from build123d import *

# Parameters (mm, degrees)
F0_W     = 28.35
F0_H     = 108.95
F0_W_2   = 6
F0_H_2   = 28
F0_W_3   = 4
F0_H_3   = 32.75
F0_H_4   = 9.8
F0_H_5   = 24
F0_W_4   = 9.65
F0_H_6   = 76.2
F0_H_7   = 11.1
F0_R     = 3
F1_DEPTH = 1


# Not quite as in the source:
# - a feature names something its author has since deleted; it is built from what else it names


with BuildPart() as f1:
    # F0 (on Right) → F1 (new body)
    with BuildSketch(Plane.YZ):
        Polygon((178.337747033, -16.9212994559), (149.987747033, -16.9212994559), (130.337747033, -16.9212994559), (130.337747033, -39.6712994559), (251.987747033, -39.6712994559), (251.987747033, -16.9212994559), (182.337747033, -16.9212994559), align=None)
        with Locations((164.162747033, 37.5537005441)):
            Rectangle(F0_W, F0_H)
        Polygon((130.337747033, -16.9212994559), (149.987747033, -16.9212994559), (149.987747033, 92.0287005441), (148.337747033, 92.0287005441), (136.337747033, 92.0287005441), (136.337747033, 68.0287005441), (136.337747033, 56.9287005441), (136.337747033, 28.9287005441), (136.337747033, 19.1287005441), (136.337747033, -8.8712994559), (130.337747033, -8.8712994559), align=None)
        Polygon((130.337747033, -39.6712994559), (130.337747033, -16.9212994559), (110.687747033, -16.9212994559), (82.337747033, -16.9212994559), (82.337747033, -28.2962994559), (82.337747033, -39.6712994559), align=None)
        Polygon((110.687747033, -16.9212994559), (130.337747033, -16.9212994559), (130.337747033, -8.8712994559), (124.337747033, -8.8712994559), (124.337747033, 19.1287005441), (124.337747033, 21.9287005441), (124.337747033, 24.7287005441), (124.337747033, 27.5287005441), (124.337747033, 28.9287005441), (124.337747033, 56.9287005441), (130.337747033, 56.9287005441), (130.337747033, 68.0287005441), (124.337747033, 68.0287005441), (124.337747033, 92.0287005441), (130.337747033, 92.0287005441), (136.337747033, 92.0287005441), (148.337747033, 92.0287005441), (148.337747033, 102.1287005441), (148.337747033, 105.1287005441), (143.337747033, 105.1287005441), (130.337747033, 105.1287005441), (112.337747033, 105.1287005441), (112.337747033, 102.1287005441), (112.337747033, 92.0287005441), (110.687747033, 92.0287005441), align=None)
        Polygon((178.337747033, 92.0287005441), (178.337747033, -16.9212994559), (182.337747033, -16.9212994559), (182.337747033, 92.0287005441), (179.8798441887, 92.0287005441), align=None)
        Polygon((82.337747033, -16.9212994559), (110.687747033, -16.9212994559), (110.687747033, 92.0287005441), (82.337747033, 92.0287005441), (82.337747033, 15.8287005441), align=None)
        with Locations((133.337747033, 5.1287005441)):
            Rectangle(F0_W_2, F0_H_2)
        with Locations((127.337747033, 5.1287005441)):
            Rectangle(F0_W_2, F0_H_2)
        Polygon((182.337747033, 92.0287005441), (182.337747033, -16.9212994559), (251.987747033, -16.9212994559), (251.987747033, 92.0287005441), (226.687747033, 92.0287005441), (216.162747033, 92.0287005441), (214.687747033, 92.0287005441), align=None)
        Polygon((82.337747033, -28.2962994559), (82.337747033, -16.9212994559), (78.337747033, -16.9212994559), (68.687747033, -16.9212994559), (68.687747033, -28.2962994559), align=None)
        with Locations((80.337747033, -0.5462994559)):
            Rectangle(F0_W_3, F0_H_3)
        with Locations((133.337747033, 24.0287005441)):
            Rectangle(F0_W_2, F0_H_4)
        Polygon((124.337747033, 19.1287005441), (130.337747033, 19.1287005441), (130.337747033, 28.9287005441), (124.337747033, 28.9287005441), (124.337747033, 27.5287005441), (124.337747033, 24.7287005441), (124.337747033, 21.9287005441), align=None)
        Polygon((60.012747033, -39.6712994559), (82.337747033, -39.6712994559), (82.337747033, -28.2962994559), (68.687747033, -28.2962994559), (63.512747033, -28.2962994559), (60.012747033, -28.2962994559), align=None)
        with Locations((133.337747033, 80.0287005441)):
            Rectangle(F0_W_2, F0_H_5)
        with Locations((73.512747033, -0.5462994559)):
            Rectangle(F0_W_4, F0_H_3)
        with Locations((80.337747033, 53.9287005441)):
            Rectangle(F0_W_3, F0_H_6)
        with Locations((133.337747033, 42.9287005441)):
            Rectangle(F0_W_2, F0_H_2)
        with Locations((127.337747033, 42.9287005441)):
            Rectangle(F0_W_2, F0_H_2)
        with Locations((127.337747033, 80.0287005441)):
            Rectangle(F0_W_2, F0_H_5)
        with Locations((133.337747033, 62.4787005441)):
            Rectangle(F0_W_2, F0_H_7)
        with BuildLine():
            Line((68.687747033, -28.2962994559), (68.687747033, -16.9212994559))
            Line((68.687747033, -16.9212994559), (68.687747033, 15.8287005441))
            Line((68.687747033, 15.8287005441), (54.687747033, 15.8287005441))
            Line((54.687747033, 15.8287005441), (44.512747033, 15.8287005441))
            Line((44.512747033, 15.8287005441), (37.687747033, 15.8287005441))
            Line((37.687747033, 15.8287005441), (8.687747033, 15.8287005441))
            Line((8.687747033, 15.8287005441), (8.687747033, -28.2962994559))
            Line((8.687747033, -28.2962994559), (25.512747033, -28.2962994559))
            ThreePointArc((25.512747033, -28.2962994559), (31.0777181904, -14.8612706134), (44.512747033, -9.2962994559))
            ThreePointArc((44.512747033, -9.2962994559), (57.9477758755, -14.8612706134), (63.512747033, -28.2962994559))
            Line((63.512747033, -28.2962994559), (68.687747033, -28.2962994559))
        make_face()
        with Locations((26.512747033, 7.8287005441)):
            Circle(F0_R, mode=Mode.SUBTRACT)
        with BuildLine():
            ThreePointArc((59.512747033, 7.8287005441), (62.512747033, 10.8287005441), (65.512747033, 7.8287005441))
            ThreePointArc((65.512747033, 7.8287005441), (62.512747033, 4.8287005441), (59.512747033, 7.8287005441))
        make_face(mode=Mode.SUBTRACT)
        Polygon((68.687747033, 15.8287005441), (78.337747033, 15.8287005441), (78.337747033, 92.0287005441), (37.687747033, 92.0287005441), (8.687747033, 92.0287005441), (8.687747033, 32.6287005441), (33.187747033, 32.6287005441), (37.687747033, 32.6287005441), (37.687747033, 15.8287005441), (44.512747033, 15.8287005441), (54.687747033, 15.8287005441), align=None)
        with BuildLine():
            ThreePointArc((44.512747033, -12.7962994559), (55.4729021414, -17.3361443475), (60.012747033, -28.2962994559))
            Line((60.012747033, -28.2962994559), (63.512747033, -28.2962994559))
            ThreePointArc((63.512747033, -28.2962994559), (57.9477758755, -14.8612706134), (44.512747033, -9.2962994559))
            Line((44.512747033, -9.2962994559), (44.512747033, -12.7962994559))
        make_face()
        with BuildLine():
            ThreePointArc((29.012747033, -28.2962994559), (33.5525919246, -17.3361443475), (44.512747033, -12.7962994559))
            Line((44.512747033, -12.7962994559), (44.512747033, -9.2962994559))
            ThreePointArc((44.512747033, -9.2962994559), (31.0777181904, -14.8612706134), (25.512747033, -28.2962994559))
            Line((25.512747033, -28.2962994559), (28.8426652551, -28.2962994559))
            Line((28.8426652551, -28.2962994559), (29.012747033, -28.2962994559))
        make_face()
        Polygon((29.012747033, -39.6712994559), (29.012747033, -28.2962994559), (28.8426652551, -28.2962994559), (25.512747033, -28.2962994559), (8.687747033, -28.2962994559), (8.687747033, -39.6712994559), align=None)
        Polygon((33.187747033, 32.6287005441), (8.687747033, 32.6287005441), (8.687747033, 15.8287005441), (37.687747033, 15.8287005441), (37.687747033, 32.6287005441), align=None)
    extrude(amount=F1_DEPTH)


solid = f1.part
Model file for the job. Use its own axes, mm. Give positions to 0.01 mm unless a question says otherwise; leave off trailing zeros. Order: outer loops, then holes, each group sorted by start corner. A loop starts at its lowest first (then second) coordinate and runs counter-clockwise, first axis right, second up. Notation, with made-up numbers: M -5.5,17 L 51.5,17 A6 cw 51.5,25 Z; hole C -2.75,72 d5. An arc over 180 degrees is marked long. Write item = value, one per line.
Q1. Cut at A-A, the plane z = -23. List the corners of the cut face in (x, y), then the cut area to 3 significant figures.
Derived:
outline = M 0,8.69 L 1,8.69 L 1,29.95 L 0,29.95 Z; M 0,59.08 L 1,59.08 L 1,251.99 L 0,251.99 Z
area = 214 mm2
Q2. Cut at C-C, the plane y = 182.5. List the corners of the cut face in (x, z).
Derived:
outline = M 0,-39.67 L 1,-39.67 L 1,92.03 L 0,92.03 Z
Q3. Drill centre lines: line 1 (Z direction, x = 0.5, y = 88.5); line 2 (Y direction, x = 0.15, z = 96.5); line 3 (Y direction, x = 0.1, z = -15). Where is each one in solid material? Low to high. Write a range as [from, to].
Derived:
line_1 = [-39.67, 92.03]
line_2 = [112.34, 148.34]
line_3 = [8.69, 36.55], [52.48, 251.99]
Q4. Cut at B-B, the plane x = 0.55. List the corners of the cut face in (y, z), then the cut area to 3 significant figures.
Derived:
outline = M 8.69,-39.67 L 29.01,-39.67 L 29.01,-28.3 A15.5 cw 60.01,-28.3 L 60.01,-39.67 L 251.99,-39.67 L 251.99,92.03 L 148.34,92.03 L 148.34,105.13 L 112.34,105.13 L 112.34,92.03 L 8.69,92.03 Z; hole C 26.51,7.83 d6; hole C 62.51,7.83 d6
area = 31,700 mm2
Q5. Flat gauge pins, fed straight in: pin 1 (0.5 mm diameter, centred on x = 0.5, z = 98.5, fed in from +Y); pin 2 (7 mm diameter, centred on y = 26.51, z = 7.83, fed in from +X); pin 3 (0.5 mm diameter, centred on x = 0.5, y = 199, fed in from +Z); pin 4 (5 mm diameter, centred on y = 62.51, z = 7.83, fed in from -X). Where does each tip first touch, or does it go through?
Derived:
pin_1 = 148.34
pin_2 = 1
pin_3 = 92.03
pin_4 = through
